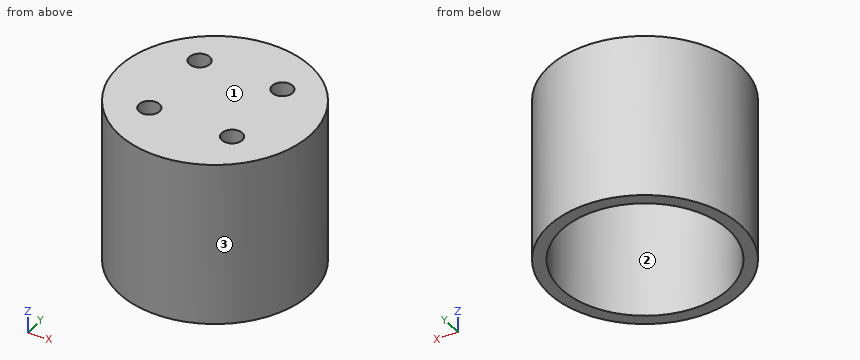
```python
from build123d import *

# Parameters (mm, degrees)
F0_R     = 7
F0_R_2   = 6.1
F1_DEPTH = 10
F2_R     = 7
F3_DEPTH = 2
F4_R     = 0.75
F5_DEPTH = 2


with BuildPart() as f1:
    # F0 (on Top) → F1 (new body)
    with BuildSketch(Plane.XY):
        Circle(F0_R)
        Circle(F0_R_2, mode=Mode.SUBTRACT)
    extrude(amount=F1_DEPTH)

    # F2 (on face) → F3 (join)
    with BuildSketch(Plane.XY.offset(10)):
        Circle(F2_R)
    extrude(amount=F3_DEPTH)

    # F4 (on face) → F5 (cut, through all)
    with BuildSketch(Plane.XY.offset(12)):
        with Locations((2.938619, -2.795266)):
            Circle(F4_R)
        with Locations((2.938619, 3.204734)):
            Circle(F4_R)
        with Locations((-3.061381, -2.795266)):
            Circle(F4_R)
        with Locations((-3.061381, 3.204734)):
            Circle(F4_R)
    extrude(amount=-F5_DEPTH, mode=Mode.SUBTRACT)


solid = f1.part
```
Model file for the job. Use its own axes, mm. Face numbers are marked on the shaded views. Give positions to 0.01 mm unless a question says otherwise; leave off trailing zeros. Write each loop counter-clockwise with the first axis right and the second up, starting at its lowest first coordinate (ties: lowest second). Pieces come first, ordered by that corner, then holes. Notation, with made-up numbers: M 88,89.25 L 144,89.25 A18 ccw 144,106.25 Z; hole C 52,58.25 d7. An arc over 180 degrees is marked long. Use a Markdown table: item, result.
1) Drill centre lines: line 1 (Y direction, x = 0, z = 4.5); line 2 (Z direction, x = -2, y = 4.5); line 3 (Y direction, x = 5.25, z = 4.5). Where is each one in solid material? Low to high. Write a range as from..to.
Responses:
| item | result |
|---|---|
| line 1 | y = -7..-6.1, 6.1..7 |
| line 2 | z = 10..12 |
| line 3 | y = -4.63..-3.11, 3.11..4.63 |
2) Pin check, flat tips, straight feed: pin 1 (2.5 mm diameter, centred on x = -3.06, y = 3.2, fed in from -Z); pin 2 (3 mm diameter, centred on x = -3, z = 6.5, fed in from -Y); pin 3 (5 mm diameter, centred on y = 3, z = 7.5, fed in from +X). Stop position of each tip, or through.
Responses:
| item | result |
|---|---|
| pin 1 | stops at z = 10 |
| pin 2 | stops at y = -6.84 |
| pin 3 | stops at x = 6.98 |
3) Cut at A-A (x = 0). List the corners of the cut face in (y, z).
Responses:
| item | result |
|---|---|
| outline | M -7,0 L -6.1,0 L -6.1,10 L 6.1,10 L 6.1,0 L 7,0 L 7,12 L -7,12 Z |
4) Cut at C-C (z = 8.5). List the corners of the cut face in (x, y), and give its area (3 significant figures).
Responses:
| item | result |
|---|---|
| outline | C 0,0 d14; hole C 0,0 d12.2 |
| area | 37.0 mm2 |
5) Pull direction Y, two halves, no side cores. Call the marked faces 1, 2 and 3: +Y half, -Y half, draft (parallel to the pull), parting line (faces both ways), or undercut.
Responses:
| item | result |
|---|---|
| face 1 | draft |
| face 2 | undercut |
| face 3 | parting line |
6) Cut at D-D (y = -2.25). List the corners of the cut face in (x, z), and give its area (3 significant figures).
Responses:
| item | result |
|---|---|
| outline | M -6.63,0 L -5.67,0 L -5.67,10 L -3.58,10 L -3.58,12 L -6.63,12 Z; M -2.55,10 L 2.42,10 L 2.42,12 L -2.55,12 Z; M 3.45,10 L 5.67,10 L 5.67,0 L 6.63,0 L 6.63,12 L 3.45,12 Z |
| area | 41.6 mm2 |
